Can you work these out from the model? Positions are in its coordinate system, mm. Face numbers are marked on the shaded views. A direction names the side the tool comes from. Give positions to 0.01 mm unless a question says otherwise; leave off trailing zeros. Write each loop counter-clockwise with the first axis right and the second up, starting at its lowest first coordinate (ties: lowest second). Pieces come first, ordered by that corner, then holes.
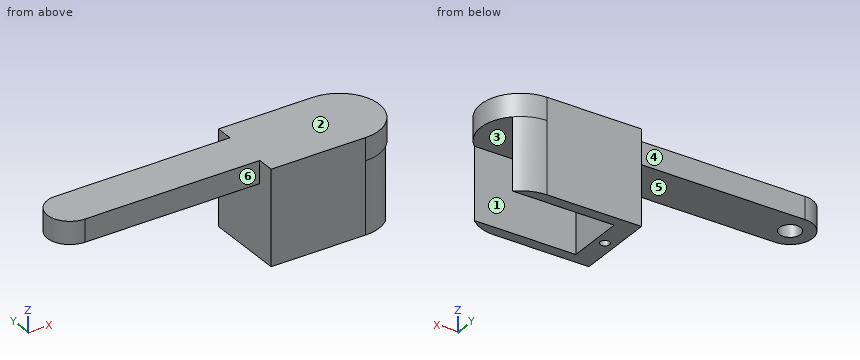
from build123d import *

# Parameters (mm, degrees)
BOSS_EXTRUDE1_DEPTH = 5
SKETCH2_R           = 2.35
CUT_EXTRUDE1_DEPTH  = 3
BOSS_EXTRUDE3_DEPTH = 5
BOSS_EXTRUDE4_DEPTH = 16
SKETCH5_R           = 1.025
CUT_EXTRUDE2_DEPTH  = 5


with BuildPart() as part:
    # Sketch1 → Boss-Extrude1 (new body)
    with BuildSketch(Plane.XY):
        with BuildLine():
            Line((0, 5), (60, 5))
            ThreePointArc((60, 5), (65, 0), (60, -5))
            Line((60, -5), (0, -5))
            ThreePointArc((0, -5), (-5, 0), (0, 5))
        make_face()
    extrude(amount=BOSS_EXTRUDE1_DEPTH)

    # Sketch2 → Cut-Extrude1 (cut)
    with BuildSketch(Plane(origin=(0, 0, 0), x_dir=(-1, 0, 0), z_dir=(0, 0, -1))):
        Circle(SKETCH2_R)
    extrude(amount=-CUT_EXTRUDE1_DEPTH, mode=Mode.SUBTRACT)

    # Sketch3 → Boss-Extrude3 (add)
    with BuildSketch(Plane.XY.offset(5)):
        with BuildLine():
            Line((38.95, -6.35), (38.95, 6.35))
            Line((38.95, 6.35), (38.95, 8.85))
            Line((38.95, 8.85), (60, 8.85))
            ThreePointArc((60, 8.85), (68.85, 0), (60, -8.85))
            Line((60, -8.85), (38.95, -8.85))
            Line((38.95, -8.85), (38.95, -6.35))
        make_face()
    extrude(amount=-BOSS_EXTRUDE3_DEPTH)

    # Sketch4 → Boss-Extrude4 (add)
    with BuildSketch(Plane(origin=(0, 0, 0), x_dir=(-1, 0, 0), z_dir=(0, 0, -1))):
        with BuildLine():
            Line((-60, 8.85), (-38.95, 8.85))
            Line((-38.95, 8.85), (-38.95, 5))
            Line((-38.95, 5), (-38.95, -5))
            Line((-38.95, -5), (-38.95, -8.85))
            Line((-38.95, -8.85), (-60, -8.85))
            ThreePointArc((-60, -8.85), (-63.258834147, -8.228152891), (-66.059702963, -6.45))
            Line((-66.059702963, -6.45), (-43.45, -6.45))
            Line((-43.45, -6.45), (-43.45, 6.45))
            Line((-43.45, 6.45), (-66.059702963, 6.45))
            ThreePointArc((-66.059702963, 6.45), (-63.258834147, 8.228152891), (-60, 8.85))
        make_face()
    extrude(amount=BOSS_EXTRUDE4_DEPTH)

    # Sketch5 → Cut-Extrude2 (cut)
    with BuildSketch(Plane(origin=(0, 0, -16), x_dir=(-1, 0, 0), z_dir=(0, 0, -1))):
        with Locations((-41.25, 0)):
            Circle(SKETCH5_R)
    extrude(amount=-CUT_EXTRUDE2_DEPTH, mode=Mode.SUBTRACT)


solid = part.part
(1) For the marked faces 1 and 2, which set-ups out of +Z, -Z, +X, -X, +Y, -Y let a thin tool reach every point of the face, with its end or its side?
Returned:
face 1: -Z, +X
face 2: +Z, +X, -X, +Y, -Y
(2) Imagine slicing it at B-B, the plane x = 49. Write out the boundary of the cut face in (y, z).
Returned:
outline: (-8.85, -16) - (-6.45, -16) - (-6.45, 0) - (6.45, 0) - (6.45, -16) - (8.85, -16) - (8.85, 5) - (-8.85, 5) - close
(3) Imagine slicing it at A-A, the plane z = 2. Write out the boundary of the cut face in (x, y), plus the area to 3 significant figures.
Returned:
outline: (0, -5) - (38.95, -5) - (38.95, -8.85) - (60, -8.85) arc R8.85 ccw to (60, 8.85) - (38.95, 8.85) - (38.95, 5) - (0, 5) arc R5 ccw to start; hole circle Ø4.7 at (0, 0)
area: 907 mm2
(4) Imagine slicing it at D-D, the plane z = -4.75. Write out the boundary of the cut face in (x, y).
Returned:
outline: (38.95, -8.85) - (60, -8.85) arc R8.85 ccw to (66.06, -6.45) - (43.45, -6.45) - (43.45, 6.45) - (66.06, 6.45) arc R8.85 ccw to (60, 8.85) - (38.95, 8.85) - close
(5) Will these pins go through, and if not, where does the flat tip stop? P1, Ø3, axis at x = 25.5, y = -2.5, coming from the -Z side; P2, Ø4, axis at y = 2.5, z = -9.5, coming from the +X side; P3, Ø5.5, axis at x = 17.5, z = 2, coming from the +Y side.
Returned:
P1: stops at z = 0
P2: stops at x = 43.45
P3: stops at y = 5
(6) Imagine slicing it at C-C, the plane y = 0. Write out the boundary of the cut face in (x, z) (3 decimals), plus the area to 3 significant figures.
Returned:
outline: (-5, 0) - (-2.35, 0) - (-2.35, 3) - (2.35, 3) - (2.35, 0) - (38.95, 0) - (38.95, -16) - (40.225, -16) - (40.225, -11) - (42.275, -11) - (42.275, -16) - (43.45, -16) - (43.45, 0) - (68.85, 0) - (68.85, 5) - (-5, 5) - close
area: 417 mm2
(7) If I drill on L1, parallel to Y at x = 53, z = -10.25; L2, parallel to Y at x = 0, z = 1.05; L3, parallel to X at y = -3.5, z = -13.25, over which ranges is the centre line in solid material (lowest first)?
Returned:
L1: y = -8.85 to -6.45, 6.45 to 8.85
L2: y = -5 to -2.35, 2.35 to 5
L3: x = 38.95 to 43.45
(8) If we mould it in two halves opening along Y, with no side actions, what happens to the marked faces 3, 4, 5 and 6? For each: +Y half, -Y half, draft (parallel to the pull), parting line (faces both ways), or undercut.
Returned:
face 3: undercut
face 4: +Y half
face 5: draft
face 6: -Y half
